The listing builds one solid part. Answer for the finished solid, in the listing's coordinates (mm). A direction names the side the tool comes from. Round coordinates to 2 decimals unless told otherwise and drop trailing zeros. Order: outer loops, then holes, each group sorted by start corner. A loop starts at its lowest first (then second) coordinate and runs counter-clockwise, first axis right, second up. Notation, with made-up numbers: M 52.25,-11.75 L 63.25,-11.75 A14 cw 63.25,-2.75 Z; hole C 44,-7.5 d7. An arc over 180 degrees is marked long. Write item = value, one per line. Start each with the question number.
(1) A cutting plane is placed at C-C, the plane x = 1326.5. Determine the outline of the cut face in (y, z), and give its area (3 significant figures).
(2) A cutting plane is placed at D-D, the plane y = -741. Determine the outline of the cut face in (x, z).
(3) For a pull along Y with two mould halves and no side action, classify faces 3 (the face through (1638, -939.698, 200)), 4 (the face through (858, -725, 406.4)), 5 (the face through (887, 76.302, 200)), 6 (the face through (858, -1549.298, 200)) as released by +Y, released by -Y, zero draft, split by the parting line, or undercut.
(4) Straight lines are drawn through the part: probe 1 along Y at (x, z) = (1573, 31); probe 2 along Y at (x, z) = (1219, 209); probe 3 along X at (y, z) = (-794.5, 134). For each, find the intervals that lie inside material, in ascending order. Write a range as from..to.
(5) Each of these flat-tipped pins is pushed along its axis until it touches: pin 1 (12 mm diameter, centred on x = 1231.5, y = -181, fed in from -Z); pin 2 (10 mm diameter, centred on y = -843, z = 332, fed in from +X). Where does it stop, or does it pass through?
(6) A cutting plane is placed at B-B, the plane z = 74.5. Determine the outline of the cut face in (x, y), and give its area (3 significant figures).
(7) A cutting plane is placed at A-A, the plane x = 1605. Determine the outline of the cut face in (y, z), and give its area (3 significant figures).
(8) Which of the six approach directions +Z, -Z, +X, -X, +Y, -Y give full straight-line access (tool end or side, diameter ignored) to faces 1 (the face through (-143.41, -725, 200)), 2 (the face through (1631, -533.298, 200))?
from build123d import *

# Parameters (mm, degrees)
F1_DEPTH = 406.4


with BuildPart() as f1:
    # F0 (on Top) → F1 (new body)
    with BuildSketch(Plane.XY):
        with BuildLine():
            Line((1888.590196, 76.302297), (-143.409804, 76.302297))
            Line((-143.409804, 76.302297), (-143.409804, -1549.297703))
            Line((-143.409804, -1549.297703), (1888.590196, -1549.297703))
            Line((1888.590196, -1549.297703), (1888.590196, -939.697703))
            Line((1888.590196, -939.697703), (1380.590196, -939.697703))
            ThreePointArc((1380.590196, -939.697703), (1177.390196, -736.497703), (1380.590196, -533.297703))
            Line((1380.590196, -533.297703), (1888.590196, -533.297703))
            Line((1888.590196, -533.297703), (1888.590196, 76.302297))
        make_face()
    extrude(amount=F1_DEPTH)


solid = f1.part
Reported:
q1.outline = M -1549.3,0 L -932.37,0 L -932.37,406.4 L -1549.3,406.4 Z; M -540.63,0 L 76.3,0 L 76.3,406.4 L -540.63,406.4 Z
q1.area = 501,000 mm²
q2.outline = M -143.41,0 L 1177.44,0 L 1177.44,406.4 L -143.41,406.4 Z
q3.face_3 = undercut
q3.face_4 = zero draft
q3.face_5 = released by +Y
q3.face_6 = released by -Y
q4.probe_1 = -1549.3..-939.7, -533.3..76.3
q4.probe_2 = -1549.3..-859.7, -613.3..76.3
q4.probe_3 = -143.41..1185.84
q5.pin_1 = 0
q5.pin_2 = 1210.72
q6.outline = M -143.41,-1549.3 L 1888.59,-1549.3 L 1888.59,-939.7 L 1380.59,-939.7 A203.2 cw 1380.59,-533.3 L 1888.59,-533.3 L 1888.59,76.3 L -143.41,76.3 Z
q6.area = 3,030,000 mm²
q7.outline = M -1549.3,0 L -939.7,0 L -939.7,406.4 L -1549.3,406.4 Z; M -533.3,0 L 76.3,0 L 76.3,406.4 L -533.3,406.4 Z
q7.area = 495,000 mm²
q8.face_1 = +Z, -Z, -X, +Y, -Y
q8.face_2 = +Z, -Z, +X
